Study the drawing (mm; zero at the part's minimum x, y, z) and answer. Round coordinates to 2 decimals unless told otherwise and drop trailing zeros. Write each loop counter-clockwise with the first axis right and the second up, starting at its lowest first coordinate (ties: lowest second). Pieces come first, ordered by that corner, then holes. Notation, with made-up numbers: (84, 89) -> (99, 89) arc R22 cw to (99, 109) -> close; hole circle Ø7 at (-13.75, 46). An arc over 180 degrees is marked (long way). Write each question's results on one line, items separated by ' | '. Start each with the question number.
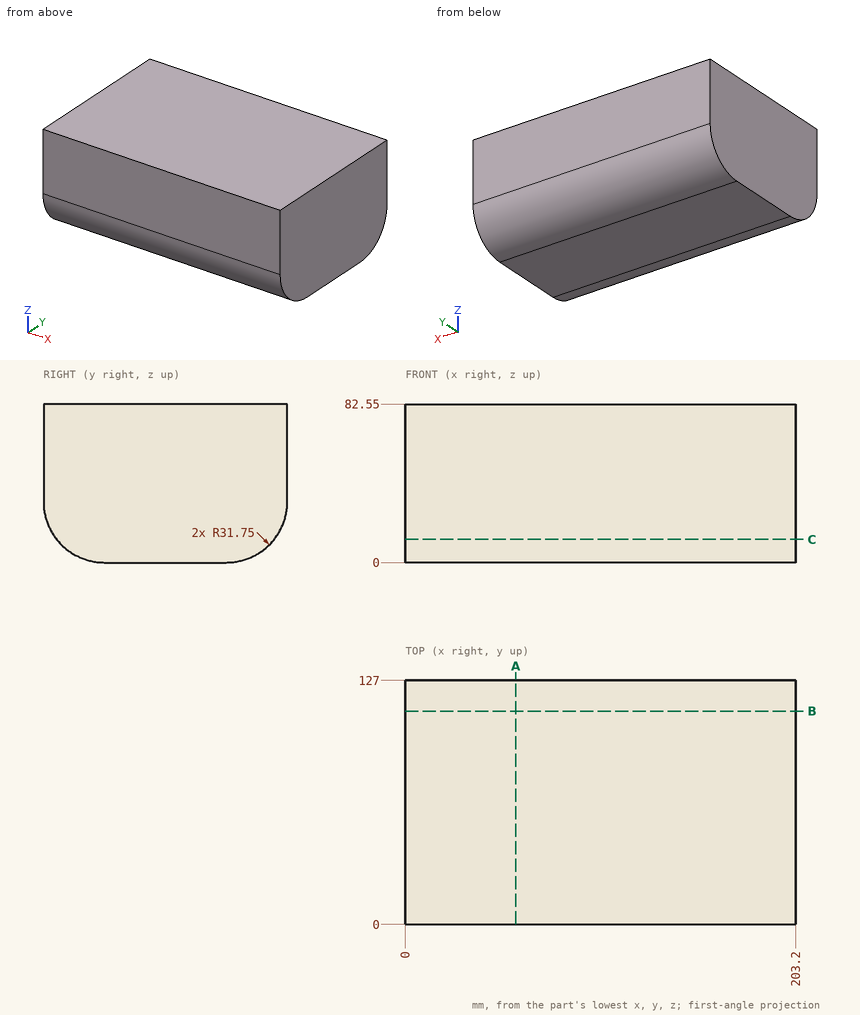
Q1. This flat-tipped pin is pushed along its axis until it touches: pin 1 (3 mm diameter, centred on x = 158, y = 55, fed in from -Z). Where does it stop, or does it pass through?
Q2. The part is cut by section A-A, the plane x = 57.5. Write down the section's boundary in (y, z), then the cut area to 3 significant figures.
Q3. The part is cut by section C-C, the plane z = 12. Write down the section's boundary in (x, y).
Q4. The part is cut by section B-B, the plane y = 111. Write down the section's boundary in (x, z), then the cut area to 3 significant figures.
Q5. Find the intervals of material crossed by line 1 (Y direction, x = 70, z = 31); line 2 (Y direction, x = 66.5, z = 18); line 3 (Z direction, x = 89, y = 111), in increasing order.
Answers follow:
1) pin 1: z = 0
2) outline: (0, 31.75) arc R31.75 ccw to (31.75, 0) -> (95.25, 0) arc R31.75 ccw to (127, 31.75) -> (127, 82.55) -> (0, 82.55) -> close | area: 10,100 mm^2
3) outline: (0, 6.89) -> (203.2, 6.89) -> (203.2, 120.11) -> (0, 120.11) -> close
4) outline: (0, 4.18) -> (203.2, 4.18) -> (203.2, 82.55) -> (0, 82.55) -> close | area: 15,900 mm^2
5) line 1: 0.01 to 126.99 | line 2: 3.13 to 123.87 | line 3: 4.18 to 82.55
